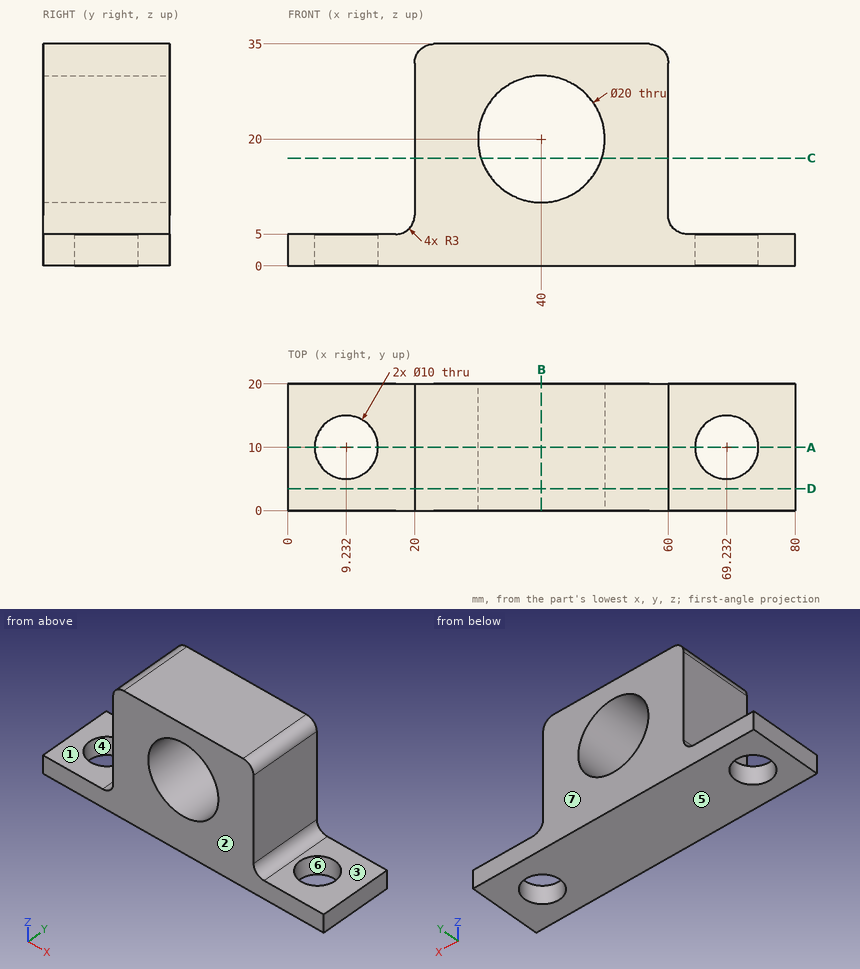
Could you check a few things on this drawing? It's one solid part, dimensions in mm from its lowest x, y, z. A direction names the side the tool comes from. Round coordinates to 2 decimals unless told otherwise and drop trailing zeros. Write each loop counter-clockwise with the first axis right and the second up, starting at its lowest first coordinate (ties: lowest second). Pieces come first, ordered by that corner, then holes. Notation, with made-up numbers: (54, -21) -> (95, -21) arc R37 cw to (95, 18) -> close; hole circle Ø1 at (7, 76). An arc over 180 degrees is marked (long way). Use a Markdown table: item, result.
1. If we section it at A-A (y = 10): List the corners of the cut face in (x, z) for me.
Answer key:
| item | result |
|---|---|
| outline | (0, 0) -> (4.23, 0) -> (4.23, 5) -> (0, 5) -> close; (14.23, 0) -> (64.23, 0) -> (64.23, 5) -> (63, 5) arc R3 cw to (60, 8) -> (60, 32) arc R3 ccw to (57, 35) -> (23, 35) arc R3 ccw to (20, 32) -> (20, 8) arc R3 cw to (17, 5) -> (14.23, 5) -> close; (74.23, 0) -> (80, 0) -> (80, 5) -> (74.23, 5) -> close; hole circle Ø20 at (40, 20) |
2. If we section it at D-D (y = 3.5): List the corners of the cut face in (x, z) for me, then the cut area to 3 significant figures.
Answer key:
| item | result |
|---|---|
| outline | (0, 0) -> (80, 0) -> (80, 5) -> (63, 5) arc R3 cw to (60, 8) -> (60, 32) arc R3 ccw to (57, 35) -> (23, 35) arc R3 ccw to (20, 32) -> (20, 8) arc R3 cw to (17, 5) -> (0, 5) -> close; hole circle Ø20 at (40, 20) |
| area | 1,290 mm^2 |
3. Which directions (+Z, -Z, +X, -X, +Y, -Y) give clear straight access to the entire face, cutting with the end or side of a thin tool? Please do the marked faces 1, 2 and 3.
Answer key:
| item | result |
|---|---|
| face 1 | +Z, -X, +Y, -Y |
| face 2 | +Z, -Z, +X, -X, -Y |
| face 3 | +Z, +X, +Y, -Y |
4. For pin 1 Ø1 at (x, z) = (31, 20) entering from -Y; pin 2 Ø6 at (y, z) = (13.5, 24.5) entering from -X; pin 3 Ø8.5 at (x, y) = (10, 6.5) entering from +Z, each with a flat end and sliding along its axis, tell me the tip position at first contact or that it passes through.
Answer key:
| item | result |
|---|---|
| pin 1 | passes through |
| pin 2 | stops at x = 20 |
| pin 3 | stops at z = 5 |
5. If we section it at B-B (x = 40): List the corners of the cut face in (y, z) for me.
Answer key:
| item | result |
|---|---|
| outline | (0, 0) -> (20, 0) -> (20, 10) -> (0, 10) -> close; (0, 30) -> (20, 30) -> (20, 35) -> (0, 35) -> close |
6. If we section it at C-C (z = 17): List the corners of the cut face in (x, y) for me.
Answer key:
| item | result |
|---|---|
| outline | (20, 0) -> (30.46, 0) -> (30.46, 20) -> (20, 20) -> close; (49.54, 0) -> (60, 0) -> (60, 20) -> (49.54, 20) -> close |
7. We'd pull the mould along Y, two halves only. Please class the marked faces 4, 5, 6 and 7: +Y half, -Y half, draft (parallel to the pull), parting line (faces both ways), or undercut.
Answer key:
| item | result |
|---|---|
| face 4 | undercut |
| face 5 | draft |
| face 6 | undercut |
| face 7 | +Y half |
8. Please list where these lines run through material, in increasing order: probe 1 along Z at (x, y) = (40, 7.75); probe 2 along Z at (x, y) = (36, 8.75) (1 decimal); probe 3 along X at (y, z) = (4.75, 25).
Answer key:
| item | result |
|---|---|
| probe 1 | z = 0 to 10, 30 to 35 |
| probe 2 | z = 0 to 10.8, 29.2 to 35 |
| probe 3 | x = 20 to 31.34, 48.66 to 60 |
